from build123d import *

# Parameters (mm, degrees)
TOP_SIDE_R                   = 0.5
BASE_MODEL_DEPTH             = 0.5
BOSS_EXTRUDE1_DEPTH          = 15
BOSS_EXTRUDE2_DEPTH          = 75
BOSS_EXTRUDE2_DEPTH_BACK     = 20
SKETCH9_W                    = 120
SKETCH9_H                    = 26
F_5_0_5_DIAMETER_HOLE1_D     = 5
CUT_EXTRUDE1_START           = 2.55
CUT_EXTRUDE1_DEPTH           = 21.3
CUT_EXTRUDE2_DEPTH           = 98.85991263
CUT_EXTRUDE2_DEPTH_BACK      = 9.8
CUT_EXTRUDE2_START           = 2.55
DRAFT11_START                = -48.5
DRAFT11_DEPTH                = 97
DRAFT11_START_2              = -52
DRAFT11_2_DEPTH              = 104
DRAFT11_START_3              = -9.867171929
DRAFT11_3_DEPTH              = 2.617171929
CUT_EXTRUDE5_START           = -18.75
CUT_EXTRUDE5_DEPTH           = 36
FILLET2_R                    = 10
CUT_EXTRUDE3_START           = 13.25
SKETCH12_R                   = 6.5
CUT_EXTRUDE3_DEPTH           = 4
CUT_EXTRUDE4_START           = 7.55
SKETCH14_R                   = 6.5
CUT_EXTRUDE4_DEPTH           = 11.2
CUT_EXTRUDE6_START           = -6.25
CUT_EXTRUDE6_DEPTH           = 25
CUT_EXTRUDE7_DEPTH           = 98.85991263
CUT_EXTRUDE7_DEPTH_BACK      = 7
CUT_EXTRUDE7_START           = 17
CUT_EXTRUDE8_START           = 17
CUT_EXTRUDE8_DEPTH           = 81.85991263
CUT_EXTRUDE9_START           = 8
CUT_EXTRUDE9_DEPTH           = 90.85991263
F_3_0_3_DIAMETER_HOLE1_D     = 3
F_3_0_3_DIAMETER_HOLE1_DEPTH = 15
F_3_0_3_DIAMETER_HOLE1_TIP   = 0.901290929


with BuildPart() as part:
    # Top Side → Base Model (new, symmetric)
    with BuildSketch(Plane(origin=(0, 0, 0), x_dir=(1, 0, 0), z_dir=(0, 1, 0))):
        with Locations(Location((0, 0, 0), (0, 0, 270))):
            Circle(TOP_SIDE_R)
    extrude(amount=BASE_MODEL_DEPTH, both=True)



with BuildPart() as body_2:
    # Sketch3 → Base (revolve)
    with BuildSketch(Plane(origin=(0, 0, 0), x_dir=(0, 0, -1), z_dir=(1, 0, 0))):
        Polygon((0, -18.75), (30, -18.75), (31.25, -17.25), (32.5, -17.25), (32.5, -14.25), (30, -14.25), (30, -9.25), (32.5, -9.25), (32.5, -7.25), (30, -7.25), (30, 18.75), (0, 18.75), align=None)
    revolve(axis=Axis((0, -18.75, 0), (0, 1, 0)))

    # Sketch8 → Boss-Extrude1 (add, symmetric)
    with BuildSketch(Plane(origin=(0, 0, 0), x_dir=(0, 0, -1), z_dir=(1, 0, 0))):
        Polygon((0, 4.25), (51.5, 4.25), (51.5, 8.25), (45.5, 13.25), (0, 13.25), align=None)
    extrude(amount=BOSS_EXTRUDE1_DEPTH, both=True)


with BuildPart() as part_1:
    add(part.part)

    add(body_2.part)  # Boss-Extrude2 merges body 2
    # Sketch9 → Boss-Extrude2 (add, two sides: drawn at the far end of the back side and taken through both)
    with BuildSketch(Plane.XY.offset(-BOSS_EXTRUDE2_DEPTH_BACK)):
        with Locations((0, 5.75)):
            Rectangle(SKETCH9_W, SKETCH9_H)
    extrude(amount=BOSS_EXTRUDE2_DEPTH + BOSS_EXTRUDE2_DEPTH_BACK)

    # Ø5.0 (5) Diameter Hole1 (through all)
    with Locations(Plane(origin=(0, 18.75, 0), x_dir=(1, 0, 0), z_dir=(0, 1, 0))):
        with Locations((-51.5, -35.2), (0, 41.034834557), (51.5, -35.2)):
            Hole(F_5_0_5_DIAMETER_HOLE1_D / 2)

    # Bottom Side Sketch5 → Cut-Extrude1 (cut)
    with BuildSketch(Plane(origin=(0, 0, 0), x_dir=(1, 0, 0), z_dir=(0, 1, 0)).offset(CUT_EXTRUDE1_START)):
        with BuildLine():
            Line((-25.617376915, 20), (-46, -6.107466904))
            Line((-46, -6.107466904), (-46, -40))
            Line((-46, -40), (-48.5, -44.330127019))
            Line((-48.5, -44.330127019), (-48.5, -65))
            Line((-48.5, -65), (-52, -65))
            Line((-52, -65), (-52, -116.5))
            Line((-52, -116.5), (-101.5, -116.5))
            Line((-101.5, -116.5), (-101.5, 101.5))
            Line((-101.5, 101.5), (101.5, 101.5))
            Line((101.5, 101.5), (101.5, -116.5))
            Line((101.5, -116.5), (52, -116.5))
            Line((52, -116.5), (52, -65))
            Line((52, -65), (48.5, -65))
            Line((48.5, -65), (48.5, -44.330127019))
            Line((48.5, -44.330127019), (46, -40))
            Line((46, -40), (46, -6.107466904))
            Line((46, -6.107466904), (25.617376915, 20))
            ThreePointArc((25.617376915, 20), (0, 32.5), (-25.617376915, 20))
        make_face()
    extrude(amount=-CUT_EXTRUDE1_DEPTH, mode=Mode.SUBTRACT)

    # Sketch11 → Cut-Extrude2 (cut, two sides: drawn at the far end of the back side and taken through both)
    with BuildSketch(Plane(origin=(0, 0, 0), x_dir=(1, 0, 0), z_dir=(0, 1, 0)).offset(CUT_EXTRUDE2_START - CUT_EXTRUDE2_DEPTH_BACK)):
        with BuildLine():
            Line((-52, -116.5), (-52, -65))
            Line((-52, -65), (-58.587704801, -44.296325315))
            ThreePointArc((-58.587704801, -44.296325315), (-59.408678786, -29.272976119), (-52.832552516, -15.740438196))
            Line((-52.832552516, -15.740438196), (-22.832552516, 19.459561804))
            ThreePointArc((-22.832552516, 19.459561804), (-19.195234326, 23.055215877), (-15, 25.980762114))
            Line((-15, 25.980762114), (-5.996666068, 47.507986456))
            ThreePointArc((-5.996666068, 47.507986456), (0, 51.5), (5.996666068, 47.507986456))
            Line((5.996666068, 47.507986456), (15, 25.980762114))
            ThreePointArc((15, 25.980762114), (19.195234326, 23.055215877), (22.832552516, 19.459561804))
            Line((22.832552516, 19.459561804), (52.832552516, -15.740438196))
            ThreePointArc((52.832552516, -15.740438196), (59.408678786, -29.272976119), (58.587704801, -44.296325315))
            Line((58.587704801, -44.296325315), (52, -65))
            Line((52, -65), (52, -116.5))
            Line((52, -116.5), (101.5, -116.5))
            Line((101.5, -116.5), (101.5, 101.5))
            Line((101.5, 101.5), (-101.5, 101.5))
            Line((-101.5, 101.5), (-101.5, -116.5))
            Line((-101.5, -116.5), (-52, -116.5))
        make_face()
    extrude(amount=CUT_EXTRUDE2_DEPTH + CUT_EXTRUDE2_DEPTH_BACK, mode=Mode.SUBTRACT)

    # Draft11: read off the stored shape, not the designer's step
    # Draft11 outline → Draft11 (add)
    with BuildSketch(Plane.YZ.offset(DRAFT11_START)):
        Polygon((-7.25, 75), (-10.216379624, 75), (-7.25, -9.945998255), align=None)
    extrude(amount=DRAFT11_DEPTH)

    # Draft11 2 outline → Draft11 2 (add)
    with BuildSketch(Plane.YZ.offset(DRAFT11_START_2)):
        Polygon((-7.25, 75), (-10.216379624, 75), (-9.867171929, 65), (-7.25, 65), align=None)
    extrude(amount=DRAFT11_2_DEPTH)

    # Draft11 3 outline → Draft11 3 (cut)
    with BuildSketch(Plane(origin=(0, 0, 0), x_dir=(1, 0, 0), z_dir=(0, 1, 0)).offset(DRAFT11_START_3)):
        Polygon((48.5, 9.945998255), (30.940703268, 9.945998255), (46, -7.723576577), (46, -40), (48.5, -44.330127019), align=None)
        Polygon((-30.940703268, 9.945998255), (-48.5, 9.945998255), (-48.5, -44.330127019), (-46, -40), (-46, -7.723576577), align=None)
    extrude(amount=DRAFT11_3_DEPTH, mode=Mode.SUBTRACT)

    # Sketch16 → Cut-Extrude5 (cut)
    with BuildSketch(Plane(origin=(0, 0, 0), x_dir=(1, 0, 0), z_dir=(0, 1, 0)).offset(CUT_EXTRUDE5_START)):
        with BuildLine():
            Line((-26.83281573, -8), (26.83281573, -8))
            ThreePointArc((26.83281573, -8), (0, 28), (-26.83281573, -8))
        make_face()
    extrude(amount=CUT_EXTRUDE5_DEPTH, mode=Mode.SUBTRACT)

    # Fillet2
    # the kernel refuses this fillet: 10 mm, written as the material it takes off along each edge
    with BuildSketch(Plane(origin=(15.887714893, 13.25, -45.5), x_dir=(0, 0, 1), z_dir=(-1, 0, 0))) as fillet2_piece_1:
        with BuildLine():
            CenterArc((FILLET2_R * 0.362049935181, -FILLET2_R), FILLET2_R, 90, 39.805571092)
            Line((-FILLET2_R * 0.278134464483, -FILLET2_R * 0.231778720403), (0, 0))
            Line((0, 0), (FILLET2_R * 0.362049935181, 0))
        make_face()
    extrude(amount=31.775429787, mode=Mode.SUBTRACT)

    # Sketch12 → Cut-Extrude3 (cut)
    with BuildSketch(Plane(origin=(0, 0, 0), x_dir=(1, 0, 0), z_dir=(0, 1, 0)).offset(CUT_EXTRUDE3_START)):
        with Locations(Location((0, 41.034834557, 0), (0, 0, 270))):
            Circle(SKETCH12_R)
    extrude(amount=-CUT_EXTRUDE3_DEPTH, mode=Mode.SUBTRACT)

    # Sketch14 → Cut-Extrude4 (cut)
    with BuildSketch(Plane(origin=(0, 0, 0), x_dir=(1, 0, 0), z_dir=(0, 1, 0)).offset(CUT_EXTRUDE4_START)):
        with Locations(Location((51.5, -35.2, 0), (0, 0, 270))):
            Circle(SKETCH14_R)
        with Locations(Location((-51.5, -35.2, 0), (0, 0, 270))):
            Circle(SKETCH14_R)
    extrude(amount=CUT_EXTRUDE4_DEPTH, mode=Mode.SUBTRACT)

    # Sketch19 → Cut-Extrude6 (cut)
    with BuildSketch(Plane(origin=(0, 0, 0), x_dir=(1, 0, 0), z_dir=(0, 1, 0)).offset(CUT_EXTRUDE6_START)):
        Polygon((35, -17), (-35, -17), (-39.5, -59.2), (-39.5, -116.5), (39.5, -116.5), (39.5, -59.2), align=None)
    extrude(amount=CUT_EXTRUDE6_DEPTH, mode=Mode.SUBTRACT)

    # Sketch20 → Cut-Extrude7 (cut, two sides: drawn at the far end of the back side and taken through both)
    with BuildSketch(Plane.XY.offset(CUT_EXTRUDE7_START - CUT_EXTRUDE7_DEPTH_BACK)):
        with BuildLine():
            Line((-25, 14.95), (25, 14.95))
            ThreePointArc((25, 14.95), (27.121320344, 14.071320344), (28, 11.95))
            Line((28, 11.95), (28, 1.75))
            ThreePointArc((28, 1.75), (27.121320344, -0.371320344), (25, -1.25))
            Line((25, -1.25), (-25, -1.25))
            ThreePointArc((-25, -1.25), (-27.121320344, -0.371320344), (-28, 1.75))
            Line((-28, 1.75), (-28, 11.95))
            ThreePointArc((-28, 11.95), (-27.121320344, 14.071320344), (-25, 14.95))
        make_face()
        with BuildLine():
            Line((-35.5, 10.35), (-35, 10.35))
            ThreePointArc((-35, 10.35), (-31.5, 6.85), (-35, 3.35))
            Line((-35, 3.35), (-35.5, 3.35))
            ThreePointArc((-35.5, 3.35), (-39, 6.85), (-35.5, 10.35))
        make_face()
        with BuildLine():
            Line((35.5, 10.35), (35, 10.35))
            ThreePointArc((35, 10.35), (31.5, 6.85), (35, 3.35))
            Line((35, 3.35), (35.5, 3.35))
            ThreePointArc((35.5, 3.35), (39, 6.85), (35.5, 10.35))
        make_face()
    extrude(amount=CUT_EXTRUDE7_DEPTH + CUT_EXTRUDE7_DEPTH_BACK, mode=Mode.SUBTRACT)

    # Sketch21 → Cut-Extrude8 (cut, through all)
    with BuildSketch(Plane.XY.offset(CUT_EXTRUDE8_START)):
        Polygon((35, 18.75), (35, 10.75), (40, 10.75), (40, 3.486117838), (46, 3.486117838), (46, -6.25), (-46, -6.25), (-46, 3.486117838), (-40, 3.486117838), (-40, 10.75), (-35, 10.75), (-35, 18.75), align=None)
    extrude(amount=CUT_EXTRUDE8_DEPTH, mode=Mode.SUBTRACT)

    # Sketch23 → Cut-Extrude9 (cut, through all)
    with BuildSketch(Plane.XY.offset(CUT_EXTRUDE9_START)):
        Polygon((-2.5, 14.95), (-25, 14.95), (-25, 12.95), (-22.25, 12.95), (-22.25, 8.85), (-25, 8.85), (-25, 4.85), (-22.25, 4.85), (-22.25, 0.75), (-25, 0.75), (-25, -1.25), (-2.5, -1.25), (-1.5, 0.75), (16, 0.75), (16, -1.25), (25, -1.25), (25, 0.75), (22.25, 0.75), (22.25, 4.85), (25, 4.85), (25, 8.85), (22.25, 8.85), (22.25, 12.95), (25, 12.95), (25, 14.95), (16, 14.95), (16, 10.75), (1.5, 10.75), (1.5, 11.95), (-1.5, 11.95), align=None)
    extrude(amount=CUT_EXTRUDE9_DEPTH, mode=Mode.SUBTRACT)

    # Ø3.0 (3) Diameter Hole1
    with Locations(Plane.XY.offset(75)):
        with Locations((-46.5, 6.85), (46.5, 6.85)):
            Hole(F_3_0_3_DIAMETER_HOLE1_D / 2, depth=F_3_0_3_DIAMETER_HOLE1_DEPTH)
            with Locations((0, 0, -(F_3_0_3_DIAMETER_HOLE1_DEPTH + F_3_0_3_DIAMETER_HOLE1_TIP / 2))):  # 118° drill point
                Cone(0, F_3_0_3_DIAMETER_HOLE1_D / 2, F_3_0_3_DIAMETER_HOLE1_TIP, mode=Mode.SUBTRACT)


solid = part_1.part
CAD build for the part. Positions are in the model's coordinates, mm. A direction names the side the tool comes from. Coordinates: 2 decimals unless noted, no trailing zeros. Write each loop counter-clockwise with the first axis right and the second up, starting at its lowest first coordinate (ties: lowest second). Pieces come first, ordered by that corner, then holes. Notation, with made-up numbers: (84.25, 10.5) - (143.25, 10.5) arc R14 cw to (143.25, 24.5) - close; hole circle Ø4 at (-18.75, 35.5). An arc over 180 degrees is marked (long way). Use a Markdown table: item, result. Add a question column.
Item 1: Flat gauge pins, fed straight in: pin 1 (5 mm diameter, centred on y = 10.5, z = 71, fed in from +X); pin 2 (6 mm diameter, centred on y = -6.5, z = -20.5, fed in from +X) (3 decimals); pin 3 (5 mm diameter, centred on y = -14, z = 12, fed in from -X); pin 4 (4.5 mm diameter, centred on x = -51.5, z = 35.2, fed in from -Y). Where does each tip first touch, or does it go through?
Item 2: 3-axis set-ups, long thin cutter, end or side, ignore diameter. For faces 1 (the face through (-45, 6.9, 67.4)), 2 (the face through (50, -4, 65)), 3 (the face through (29, -14.25, -9)), 4 (the face through (-9.76, -8.46, -31)): which of +Z, -Z, +X, -X, +Y, -Y reach the whole face in a straight line?
Item 3: Drill centre lines: L1, parallel to X at y = 6.85, z = 72.25; L2, parallel to X at y = 4.75, z = 35.2; L3, parallel to X at y = -3, z = 64.5. Where is each one in solid material? Low to high. Write a range as from..to.
Item 4: Band-saw the part on A-A, the plane z = 19. Give the number of separate pieces and of enclosed holes in the cut face, and give its area (3 significant figures).
Item 5: Mould opens along Y. For faces 5 (the face through (0.04, 11.34, -47.76)), 6 (the face through (-46, -1, 58)), 7 (the face through (-47.27, -3.38, 42.2)) say: pulls with the +Y half, pulls with the -Y half, needs draft (parallel to the pull), parting line crosses it, or undercut.
Item 6: Band-saw the part on B-B, the plane z = 0. Give the cut face in (x, y), and give its area (3 significant figures).
Numbers:
| question | item | result |
|---|---|---|
| 1 | pin 1 | x = 52 |
| 1 | pin 2 | x = 27.325 |
| 1 | pin 3 | x = -31.08 |
| 1 | pin 4 | through |
| 2 | face 1 | +Z |
| 2 | face 2 | -Z, +X, -Y |
| 2 | face 3 | none |
| 2 | face 4 | -Y |
| 3 | L1 | -52..-48, -45..-40, 40..45, 48..52 |
| 3 | L2 | -60..-54, -49..-40, 40..49, 54..60 |
| 3 | L3 | -48.5..-46, 46..48.5 |
| 4 | separate pieces | 3 |
| 4 | enclosed holes | 0 |
| 4 | area | 1,260 mm2 |
| 5 | face 5 | pulls with the +Y half |
| 5 | face 6 | undercut |
| 5 | face 7 | needs draft |
| 6 | outline | (-39.42, -7.6) - (-32.5, -7.6) - (-32.5, -9.25) - (-30, -9.25) - (-30, -14.25) - (-32.5, -14.25) - (-32.5, -17.25) - (-31.25, -17.25) - (-30, -18.75) - (-28, -18.75) - (-28, 17.25) - (28, 17.25) - (28, -18.75) - (30, -18.75) - (31.25, -17.25) - (32.5, -17.25) - (32.5, -14.25) - (30, -14.25) - (30, -9.25) - (32.5, -9.25) - (32.5, -7.6) - (39.42, -7.6) - (39.42, 18.75) - (-39.42, 18.75) - close |
| 6 | area | 755 mm2 |
